Part model, mm, in its own coordinate system. A direction names the side the tool comes from. Give positions to 0.01 mm unless a question says otherwise; leave off trailing zeros. Write each loop counter-clockwise with the first axis right and the second up, starting at its lowest first coordinate (ties: lowest second). Pieces come first, ordered by that corner, then holes.
Autodesk Inventor part; units mm, degrees
ref_plane "YZ Plane" through (0, 0, 0) normal (1, 0, 0) x (0, 1, 0)
ref_plane "XZ Plane" through (0, 0, 0) normal (0, 1, 0) x (-1, 0, 0)
ref_plane "XY Plane" through (0, 0, 0) normal (0, 0, 1) x (1, 0, 0)
sketch "草图1" plane through (0, 0, 0) normal (0, 0, 1) x (1, 0, 0)
  line L0 (15, -7.5) -> (-15, -7.5)
  line L1 (-15, -7.5) -> (-15, 7.5)
  line L2 (-15, 7.5) -> (15, 7.5)
  line L3 (15, 7.5) -> (15, -7.5)
  line L4 (15, -7.5) -> (-15, 7.5) construction
  line L5 (-15, -7.5) -> (15, 7.5) construction
  line L6 (14, 6.5) -> (-14, 6.5)
  line L7 (-14, 6.5) -> (-14, -6.5)
  line L8 (-14, -6.5) -> (14, -6.5)
  line L9 (14, -6.5) -> (14, 6.5)
  point P0 (0, 0)
  dimension "d0" = 30
  dimension "d1" = 15
  dimension "d2" = 1
extrude "拉伸1" add sketch "草图1" along normal blind 150
sketch "草图2" plane through (-15, -7.5, 0) normal (0, -1, 0) x (1, 0, 0)
  line L0 (-150, 0) -> (30, 0)
  line L1 (30, 30) -> (30, 0)
  line L2 (-150, 30) -> (30, 30)
  line L3 (-150, 30) -> (-150, 0)
  circle A0 centre (7, 7) radius 1.35
  circle A1 centre (23, 7) radius 1.35
  circle A2 centre (23, 23) radius 1.35
  circle A3 centre (-109, 7) radius 1.35
  circle A4 centre (7, 23) radius 1.35
  circle A5 centre (-127, 23) radius 1.35
  circle A6 centre (-127, 7) radius 1.35
  circle A7 centre (-143, 7) radius 1.35
  circle A8 centre (-11, 23) radius 1.35
  circle A9 centre (-11, 7) radius 1.35
  circle A10 centre (-109, 23) radius 1.35
  circle A11 centre (-143, 23) radius 1.35
  point P0 (15, 0)
extrude "拉伸2" cut sketch "草图2" against normal blind 23.75 contours A0 | A1 | A2 | A4
sketch "草图3" plane through (-15, -7.5, 0) normal (-1, 0, 0) x (0, 0, 1)
  line L0 (0, 0) -> (0, 15)
  line L1 (0, 10.637) -> (33.403, 0)
  line L2 (0, 0) -> (150, 0)
  point P0 (0, 7.5)
extrude "拉伸3" cut sketch "草图3" against normal blind 35
properties part number "40x15"
1) Saw through at D-D, the plane z = 81. Write the cut outline in (x, y).
Answers follow:
outline: (-15, -7.5) - (15, -7.5) - (15, 7.5) - (-15, 7.5) - close; hole (-14, -6.5) - (14, -6.5) - (14, 6.5) - (-14, 6.5) - close
2) Saw through at A-A, the plane x = -12.75. Write the cut outline in (y, z), then the cut area to 3 significant figures.
Answers follow:
outline: (-7.5, 33.4) - (-6.5, 30.26) - (-6.5, 150) - (-7.5, 150) - close; (6.5, 0) - (7.5, 0) - (7.5, 150) - (6.5, 150) - close
area: 268 mm2
3) Two-plate mould, pull along X, no slides. Class faces 3 (the face through (-14, 0, 74)), 4 (the face through (15, 0, 74)), 5 (the face through (-7.274, 6.993, 8.138)), 6 (the face through (0, 7.5, 74)): +X half, -X half, draft (parallel to the pull), parting line (faces both ways), or undercut.
Answers follow:
face 3: undercut
face 4: +X half
face 5: undercut
face 6: draft
4) Saw through at C-C, the plane y = -1. Write the cut outline in (x, z), then the cut area to 3 significant figures.
Answers follow:
outline: (-15, 12.99) - (-14, 12.99) - (-14, 150) - (-15, 150) - close; (14, 12.99) - (15, 12.99) - (15, 150) - (14, 150) - close
area: 274 mm2
5) Wall check: L1, parallel to Z at x = 8, y = 7.05; L2, parallel to X at y = 3.5, z = 40.5; L3, parallel to Y at x = -13.25, z = 121. Give the ranges that are in metal, low to high.
Answers follow:
L1: z = 0 to 5.65, 8.35 to 21.65, 24.35 to 150
L2: x = -15 to -14, 14 to 15
L3: y = -7.5 to -6.5, 6.5 to 7.5
6) 3-axis set-ups, long thin cutter, end or side, ignore diameter. For faces 1 (the face through (0, 6.5, 74)), 2 (the face through (9.247, 6.993, 22.483)): which of +Z, -Z, +X, -X, +Y, -Y reach the whole face in a straight line?
Answers follow:
face 1: +Z, -Z
face 2: +Y, -Y
7) Pin check, flat tip, straight feed: pin 1 Ø3 at (x, z) = (8, 23) entering from -Y. Stop position of the tip, or through.
Answers follow:
pin 1: stops at y = 6.5
8) Saw through at B-B, the plane z = 7. Write the cut outline in (x, y).
Answers follow:
outline: (-15, 0.91) - (-14, 0.91) - (-14, 6.5) - (-9.35, 6.5) - (-9.35, 7.5) - (-15, 7.5) - close; (-6.65, 6.5) - (6.65, 6.5) - (6.65, 7.5) - (-6.65, 7.5) - close; (9.35, 6.5) - (14, 6.5) - (14, 0.91) - (15, 0.91) - (15, 7.5) - (9.35, 7.5) - close
